from build123d import *

# Parameters (mm, degrees)
SKETCH1_W           = 105
SKETCH1_H           = 48
SKETCH1_R           = 6
SKETCH1_R_2         = 9
SKETCH1_R_3         = 4
BOSS_EXTRUDE1_DEPTH = 5
FILLET1_R           = 2


with BuildPart() as part:
    # Sketch1 → Boss-Extrude1 (new body)
    with BuildSketch(Plane(origin=(0, 0, 0), x_dir=(1, 0, 0), z_dir=(0, 1, 0))):
        with Locations((52.5, 24)):
            Rectangle(SKETCH1_W, SKETCH1_H)
        with Locations(Location((10, 10, 0), (0, 0, 270))):
            Circle(SKETCH1_R, mode=Mode.SUBTRACT)
        with Locations(Location((10, 38, 0), (0, 0, 270))):
            Circle(SKETCH1_R, mode=Mode.SUBTRACT)
        with Locations(Location((25, 24, 0), (0, 0, 270))):
            Circle(SKETCH1_R_2, mode=Mode.SUBTRACT)
        with Locations(Location((93, 15, 0), (0, 0, 270))):
            Circle(SKETCH1_R_3, mode=Mode.SUBTRACT)
        with Locations(Location((93, 33, 0), (0, 0, 270))):
            Circle(SKETCH1_R_3, mode=Mode.SUBTRACT)
        with BuildLine():
            Line((61.5, 33), (61.5, 15))
            ThreePointArc((61.5, 15), (65.5, 11), (69.5, 15))
            Line((69.5, 15), (69.5, 33))
            ThreePointArc((69.5, 33), (65.5, 37), (61.5, 33))
        make_face(mode=Mode.SUBTRACT)
    extrude(amount=BOSS_EXTRUDE1_DEPTH)

    # Fillet1
    fillet1_edges = [part.edges().sort_by_distance(p)[0] for p in [
        (0, 2.5, -48),
        (105, 2.5, -48),
        (105, 2.5, 0),
        (0, 2.5, 0),
    ]]
    fillet(fillet1_edges, radius=FILLET1_R)


solid = part.part
Work out the finished part from the listing and answer in its coordinate system (mm). A direction names the side the tool comes from. Give positions to 0.01 mm unless a question says otherwise; leave off trailing zeros. Write each loop counter-clockwise with the first axis right and the second up, starting at its lowest first coordinate (ties: lowest second). Pieces come first, ordered by that corner, then holes. Notation, with made-up numbers: (-25.75, 67) - (-5.75, 67) arc R21 ccw to (-5.75, 72) - close; hole circle Ø2 at (-17.75, -17). An arc over 180 degrees is marked (long way). One line per item, written item: value. Start each with the question number.
1. For a pull along Z with two mould halves and no side action, classify faces 3 (the flat face through (52, 2, 0)), 4 (the cylindrical face through (89.095, 2.465, -33.867)), 5 (the flat face through (52, 0, -24)) as +Z half, -Z half, draft (parallel to the pull), parting line (faces both ways), or undercut.
2. For faces 1 (the flat face through (61.5, 2, -24)), 2 (the cylindrical face through (0.57, 2.54, -0.6)), determine the directions among +Z, -Z, +X, -X, +Y, -Y from which every point of the face is accessible in a straight line to the end or side of a thin tool.
3. Given pin 1 (14 mm diameter, centred on x = 10, z = -10, fed in from -Y); pin 2 (5 mm diameter, centred on x = 93, z = -15, fed in from -Y), each flat-ended and moving along its own axis, determine where each tip first touches the part or whether it passes through.
4. Find section D-D (x = 25). Write down the section's boundary in (y, z).
5. Find section A-A (z = -38). Write down the section's boundary in (x, y), then the cut area to 3 significant figures.
6. Consider probe 1 along X at (y, z) = (1, -10); probe 2 along Z at (x, y) = (90.5, 0.3); probe 3 along X at (y, z) = (4.8, -21.5). Determine where each line is inside the solid, lowest interval first.
7. Find section C-C (x = 93). Write down the section's boundary in (y, z), then the cut area to 3 significant figures.
8. Find section B-B (y = 1.05). Write down the section's boundary in (x, z), then the cut area to 3 significant figures.
Geometry results:
1. face 3: +Z half
1. face 4: undercut
1. face 5: draft
2. face 1: +Y, -Y
2. face 2: +Z, -X, +Y, -Y
3. pin 1: y = 0
3. pin 2: through
4. outline: (0, -48) - (5, -48) - (5, -33) - (0, -33) - close; (0, -15) - (5, -15) - (5, 0) - (0, 0) - close
5. outline: (0, 0) - (4, 0) - (4, 5) - (0, 5) - close; (16, 0) - (105, 0) - (105, 5) - (16, 5) - close
5. area: 465 mm2
6. probe 1: 0 to 4, 16 to 105
6. probe 2: -48 to -36.12, -29.88 to -18.12, -11.88 to 0
6. probe 3: 0 to 16.35, 33.65 to 61.5, 69.5 to 105
7. outline: (0, -48) - (5, -48) - (5, -37) - (0, -37) - close; (0, -29) - (5, -29) - (5, -19) - (0, -19) - close; (0, -11) - (5, -11) - (5, 0) - (0, 0) - close
7. area: 160 mm2
8. outline: (0, -46) arc R2 ccw to (2, -48) - (103, -48) arc R2 ccw to (105, -46) - (105, -2) arc R2 ccw to (103, 0) - (2, 0) arc R2 ccw to (0, -2) - close; hole circle Ø12 at (10, -38); hole circle Ø12 at (10, -10); hole circle Ø18 at (25, -24); hole (61.5, -33) arc R4 ccw to (69.5, -33) - (69.5, -15) arc R4 ccw to (61.5, -15) - close; hole circle Ø8 at (93, -33); hole circle Ø8 at (93, -15)
8. area: 4,260 mm2
